```python
from build123d import *

# Parameters (mm, degrees)
F0_W     = 63.8
F0_H     = 47.8
F1_DEPTH = 3.2
F2_R     = 2.4
F3_DEPTH = 1.6
F6_DEPTH = 15.9
F8_R     = 1.6
F9_DEPTH = 32


with BuildPart() as f1:
    # F0 (on Top) → F1 (new body)
    with BuildSketch(Plane.XY):
        Rectangle(F0_W, F0_H)
    extrude(amount=F1_DEPTH)

    # F2 (on face) → F3 (join)
    with BuildSketch(Plane.XY.offset(3.2)):
        with Locations((-28, 20)):
            Circle(F2_R)
        with Locations((-28, 12)):
            Circle(F2_R)
        with Locations((-28, 4)):
            Circle(F2_R)
        with Locations((-28, -4)):
            Circle(F2_R)
        with Locations((-28, -12)):
            Circle(F2_R)
        with Locations((-28, -20)):
            Circle(F2_R)
        with Locations((-20, 20)):
            Circle(F2_R)
        with Locations((-20, 12)):
            Circle(F2_R)
        with Locations((-20, 4)):
            Circle(F2_R)
        with Locations((-20, -4)):
            Circle(F2_R)
        with Locations((-20, -12)):
            Circle(F2_R)
        with Locations((-20, -20)):
            Circle(F2_R)
        with Locations((-12, 20)):
            Circle(F2_R)
        with Locations((-12, 12)):
            Circle(F2_R)
        with Locations((-12, 4)):
            Circle(F2_R)
        with Locations((-12, -4)):
            Circle(F2_R)
        with Locations((-12, -12)):
            Circle(F2_R)
        with Locations((-12, -20)):
            Circle(F2_R)
        with Locations((-4, 20)):
            Circle(F2_R)
        with Locations((-4, 12)):
            Circle(F2_R)
        with Locations((-4, 4)):
            Circle(F2_R)
        with Locations((-4, -4)):
            Circle(F2_R)
        with Locations((-4, -12)):
            Circle(F2_R)
        with Locations((-4, -20)):
            Circle(F2_R)
        with Locations((4, 20)):
            Circle(F2_R)
        with Locations((4, 12)):
            Circle(F2_R)
        with Locations((4, 4)):
            Circle(F2_R)
        with Locations((4, -4)):
            Circle(F2_R)
        with Locations((4, -12)):
            Circle(F2_R)
        with Locations((4, -20)):
            Circle(F2_R)
        with Locations((12, 20)):
            Circle(F2_R)
        with Locations((12, 12)):
            Circle(F2_R)
        with Locations((12, 4)):
            Circle(F2_R)
        with Locations((12, -4)):
            Circle(F2_R)
        with Locations((12, -12)):
            Circle(F2_R)
        with Locations((12, -20)):
            Circle(F2_R)
        with Locations((20, 20)):
            Circle(F2_R)
        with Locations((20, 12)):
            Circle(F2_R)
        with Locations((20, 4)):
            Circle(F2_R)
        with Locations((20, -4)):
            Circle(F2_R)
        with Locations((20, -12)):
            Circle(F2_R)
        with Locations((20, -20)):
            Circle(F2_R)
        with Locations((28, 20)):
            Circle(F2_R)
        with Locations((28, 12)):
            Circle(F2_R)
        with Locations((28, 4)):
            Circle(F2_R)
        with Locations((28, -4)):
            Circle(F2_R)
        with Locations((28, -12)):
            Circle(F2_R)
        with Locations((28, -20)):
            Circle(F2_R)
    extrude(amount=F3_DEPTH)

    # F7: F6 across plane


with BuildPart() as f6:
    # F5 (on face) → F6 (new body, through all)
    with BuildSketch(Plane.YZ.offset(31.9)):
        with BuildLine():
            ThreePointArc((27.1, -3.2), (26.1627416998, -0.9372583002), (23.9, 0))
            Line((23.9, 0), (-23.9, 0))
            ThreePointArc((-23.9, 0), (-26.1627416998, -0.9372583002), (-27.1, -3.2))
            ThreePointArc((-27.1, -3.2), (-26.1627416998, -5.4627416998), (-23.9, -6.4))
            Line((-23.9, -6.4), (23.9, -6.4))
            ThreePointArc((23.9, -6.4), (26.1627416998, -5.4627416998), (27.1, -3.2))
        make_face()
    extrude(amount=-F6_DEPTH)


with BuildPart() as f1_1:
    add(f1.part)
    add(f6.part.mirror(Plane.YZ))


    add(f6.part)  # F9 merges F6
    # F8 (on face) → F9 (join, through all)
    with BuildSketch(Plane(origin=(16, 0, 0), x_dir=(0, -1, 0), z_dir=(-1, 0, 0))):
        with Locations((-23.9, -3.2)):
            Circle(F8_R)
        with Locations((23.9, -3.2)):
            Circle(F8_R)
        with BuildLine():
            Line((20.7, 0), (-20.7, 0))
            Line((-20.7, 0), (-11.8153602589, -8.8846397411))
            ThreePointArc((-11.8153602589, -8.8846397411), (-10.0130899865, -9.7885944374), (-8.0280111082, -9.4353606981))
            ThreePointArc((-8.0280111082, -9.4353606981), (0, -7.4), (8.0280111082, -9.4353606981))
            ThreePointArc((8.0280111082, -9.4353606981), (10.0130899865, -9.7885944374), (11.8153602589, -8.8846397411))
            Line((11.8153602589, -8.8846397411), (20.7, 0))
        make_face()
    extrude(amount=F9_DEPTH)


solid = f1_1.part
```
Model file for the job. Use its own axes, mm. A direction names the side the tool comes from. Round coordinates to 2 decimals unless told otherwise and drop trailing zeros. Write each loop counter-clockwise with the first axis right and the second up, starting at its lowest first coordinate (ties: lowest second). Pieces come first, ordered by that corner, then holes. Notation, with made-up numbers: (-36.75, 49.5) - (-19.75, 49.5) arc R15 ccw to (-19.75, 60.5) - close; hole circle Ø2 at (64.5, 88.5). An arc over 180 degrees is marked (long way). Use CSV: the item, a comma, the result in double quotes. Start each with the question number.
Item 1: Pin check, flat tips, straight feed: P1, Ø5, axis at x = -8.5, z = -2, coming from the +Y side; P2, Ø1, axis at x = 14.5, z = 2, coming from the +Y side; P3, Ø1, axis at y = 6, z = -9, coming from the -X side. Stop position of each tip, or through.
Item 2: Tool access for faces 1 (the face through (30.29, -11.28, 3.99)), 2 (the face through (0, -22, 0)), 3 (the face through (0, 22, 0)), 4 (the face through (0.224, -25.426, -2.719)): list every direction of +Z, -Z, +X, -X, +Y, -Y with a clear straight run to the whole face (end or side of a thin tool).
Item 3: Drill centre lines: L1, parallel to Y at x = 14, z = -3; L2, parallel to Y at x = 2.5, z = -3.25; L3, parallel to X at y = 18, z = -3.25. Where is each one in solid material? Low to high. Write a range as [from, to].
Item 4: Band-saw the part on C-C (x = 12). State how many separate pieces and enclosed holes the cut face has, and give its area (3 significant figures).
Item 5: Band-saw the part on B-B (z = 1.5). Write the cut outline in (x, y), and give its area (3 significant figures).
Item 6: Two-plate mould, pull along X, no slides. Class faces 5 (the face through (21.29, 6.024, 3.989)), 6 (the face through (31.9, 0, -2)), 7 (the face through (0.224, -9.985, -9.793)): released by +X, released by -X, zero draft, split by the parting line, or undercut.
Checked values:
1,P1,"stops at y = 25.5"
1,P2,"stops at y = 23.9"
1,P3,"stops at x = -16"
2,face 1,"+Z"
2,face 2,"-Y"
2,face 3,"+Y"
2,face 4,"none"
3,L1,"y = [-25.49, -22.31], [-17.7, 17.7], [22.31, 25.49]"
3,L2,"y = [-25.5, -22.3], [-17.45, 17.45], [22.3, 25.5]"
3,L3,"x = [-31.9, -16], [16, 31.9]"
4,separate pieces,"3"
4,enclosed holes,"0"
4,area,"496 mm²"
5,outline,"(-31.9, -23.9) - (31.9, -23.9) - (31.9, 23.9) - (-31.9, 23.9) - close"
5,area,"3,050 mm²"
6,face 5,"undercut"
6,face 6,"released by +X"
6,face 7,"zero draft"
